For this review, take the finished solid that the model builds, in its own axes (mm). Face numbers are marked on the shaded views. A direction names the side the tool comes from. Coordinates: 2 decimals unless noted, no trailing zeros. Loops run counter-clockwise (first coordinate to the right, second up) from the corner with the lowest first, then second, coordinate; pieces in that order, holes last.
1. Take a section at A-A, the plane y = 53. State the section outline as (x, z) points, then the cut area to 3 significant figures.
2. Mouldability with a two-part tool opening along X and no side actions: class the marked faces 1, 2 and 3 as pulls with the +X half, pulls with the -X half, needs draft (parallel to the pull), parting line crosses it, or undercut.
3. To check wall thickness, follow probe 1 along Z at (x, y) = (109.65, 70); probe 2 along X at (y, z) = (27, -32.5); probe 3 along Z at (x, y) = (109, 70). State the ranges of each line that lie inside material, in increasing order.
4. Take a section at B-B, the plane z = -23.5. State the section outline as (x, y) points.
5. Take a section at C-C, the plane y = 43. State the section outline as (x, z) points.
6. Clearance check with flat-ended pins moving along their axes: P1, Ø4, axis at y = 70, z = -130, coming from the -X side; P2, Ø3, axis at x = 67, y = 49.5, coming from the -Z side; P3, Ø2.5, axis at y = 70, z = -130, coming from the -X side. State where each tip first meets the part, or that it passes through.
7. Take a section at D-D, the plane x = 36. State the section outline as (y, z) points.
8. Machinability: for the marked faces 4 and 5, which of the approach directions +Z, -Z, +X, -X, +Y, -Y give a long, thin tool a straight path to every point of the face, cutting with its end or side? Answer none if there is none.
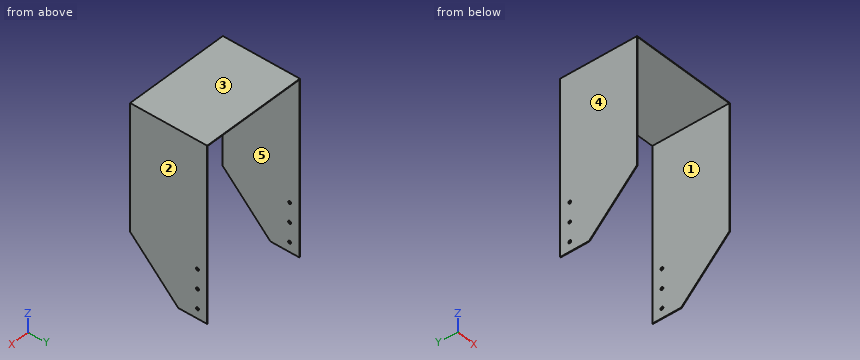
```python
from build123d import *

# Parameters (mm, degrees)
SKETCH1_W           = 110
SKETCH1_H           = 180
BOSS_EXTRUDE1_DEPTH = 80
SKETCH2_W           = 108.6
SKETCH2_H           = 179.3
CUT_EXTRUDE1_DEPTH  = 226.610283454
SKETCH4_R           = 1.5
CUT_EXTRUDE3_DEPTH  = 226.610283454
CUT_EXTRUDE5_DEPTH  = 226.610283454


with BuildPart() as part:
    # Sketch1 → Boss-Extrude1 (new body)
    with BuildSketch(Plane(origin=(0, 0, 0), x_dir=(1, 0, 0), z_dir=(0, 1, 0))):
        with Locations((55, 90)):
            Rectangle(SKETCH1_W, SKETCH1_H)
    extrude(amount=BOSS_EXTRUDE1_DEPTH)

    # Sketch2 → Cut-Extrude1 (cut, through all)
    with BuildSketch(Plane(origin=(0, 80, 0), x_dir=(1, 0, 0), z_dir=(0, 1, 0))):
        with Locations((55, 90.35)):
            Rectangle(SKETCH2_W, SKETCH2_H)
    extrude(amount=-CUT_EXTRUDE1_DEPTH, mode=Mode.SUBTRACT)

    # Sketch4 → Cut-Extrude3 (cut, through all)
    with BuildSketch(Plane(origin=(110, 0, 0), x_dir=(0, 0, -1), z_dir=(1, 0, 0))):
        with Locations((170, 70)):
            Circle(SKETCH4_R)
        with Locations((130, 70)):
            Circle(SKETCH4_R)
        with Locations((150, 70)):
            Circle(SKETCH4_R)
    extrude(amount=-CUT_EXTRUDE3_DEPTH, mode=Mode.SUBTRACT)

    # Sketch8 → Cut-Extrude5 (cut, through all)
    with BuildSketch(Plane(origin=(110, 0, 0), x_dir=(0, 0, -1), z_dir=(1, 0, 0))):
        Polygon((180, 50), (130, 0), (180, 0), align=None)
    extrude(amount=-CUT_EXTRUDE5_DEPTH, mode=Mode.SUBTRACT)


solid = part.part
```
Results list:
1. outline: (0, -180) - (0.7, -180) - (0.7, -0.7) - (109.3, -0.7) - (109.3, -180) - (110, -180) - (110, 0) - (0, 0) - close
1. area: 328 mm2
2. face 1: undercut
2. face 2: pulls with the +X half
2. face 3: needs draft
3. probe 1: z = -180 to -171.5, -168.5 to -151.5, -148.5 to -131.5, -128.5 to 0
3. probe 2: x = 0 to 0.7, 109.3 to 110
3. probe 3: z = -0.7 to 0
4. outline: (0, 0) - (0.7, 0) - (0.7, 80) - (0, 80) - close; (109.3, 0) - (110, 0) - (110, 80) - (109.3, 80) - close
5. outline: (0, -173) - (0.7, -173) - (0.7, -0.7) - (109.3, -0.7) - (109.3, -173) - (110, -173) - (110, 0) - (0, 0) - close
6. P1: stops at x = 0
6. P2: stops at z = -0.7
6. P3: passes through
7. outline: (0, -0.7) - (80, -0.7) - (80, 0) - (0, 0) - close
8. face 4: +Z, -Z, -X, +Y, -Y
8. face 5: -Z, +Y, -Y
